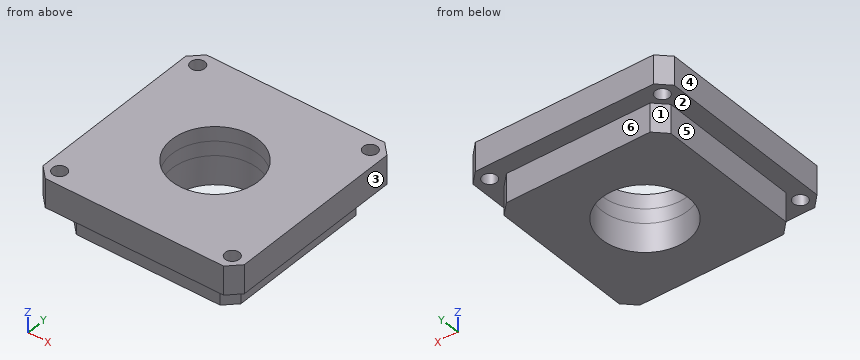
Autodesk Inventor part; units mm, degrees
ref_plane "YZ Plane" through (0, 0, 0) normal (1, 0, 0) x (0, 1, 0)
ref_plane "XZ Plane" through (0, 0, 0) normal (0, 1, 0) x (-1, 0, 0)
ref_plane "XY Plane" through (0, 0, 0) normal (0, 0, 1) x (1, 0, 0)
sketch "Sketch5" plane through (0, 0, 0) normal (0, 0, 1) x (1, 0, 0)
  circle A0 centre (15, -15) radius 1.2295
  circle A1 centre (-15, 15) radius 1.2295
  circle A2 centre (15, 15) radius 1.2295
  circle A3 centre (-15, -15) radius 1.2295
  line L0 (-15.5, -17.5) -> (-17.5, -15.5)
  line L1 (-15.5, -17.5) -> (15.5, -17.5)
  line L2 (17.5, -15.5) -> (15.5, -17.5)
  line L3 (17.5, -15.5) -> (17.5, 15.5)
  line L4 (15.5, 17.5) -> (17.5, 15.5)
  line L5 (15.5, 17.5) -> (-15.5, 17.5)
  line L6 (-17.5, 15.5) -> (-15.5, 17.5)
  line L7 (-17.5, 15.5) -> (-17.5, -15.5)
  circle A4 centre (0, 0) radius 7.5
  dimension "d59" = 15
extrude "Extrusion4" add sketch "Sketch5" against normal mid plane 5
sketch "Sketch6" plane through (0, 0, -2.5) normal (0, 0, -1) x (-1, 0, 0)
  line L0 (14.5, 12.5) -> (14.5, -12.5)
  line L1 (12.5, 14.5) -> (14.5, 12.5)
  line L2 (-12.5, 14.5) -> (12.5, 14.5)
  line L3 (-14.5, 12.5) -> (-12.5, 14.5)
  line L4 (-14.5, -12.5) -> (-14.5, 12.5)
  line L5 (-12.5, -14.5) -> (-14.5, -12.5)
  line L6 (12.5, -14.5) -> (-12.5, -14.5)
  line L7 (14.5, -12.5) -> (12.5, -14.5)
  circle A0 centre (0, 0) radius 7.5
extrude "Extrusion5" add sketch "Sketch6" along normal blind 5
properties part number "Front cover for servo motor 250 W" material "PBT Plastic"
The model under review builds one solid part; all positions refer to its coordinate system, in mm. Face numbers are marked on the shaded views. A direction names the side the tool comes from. Round coordinates to 2 decimals unless told otherwise and drop trailing zeros. Order: outer loops, then holes, each group sorted by start corner. A loop starts at its lowest first (then second) coordinate and runs counter-clockwise, first axis right, second up. Notation, with made-up numbers: (4.5, -36) -> (49.5, -36) arc R16 cw to (49.5, -27) -> close; hole circle Ø7 at (15.25, 35). An arc over 180 degrees is marked (long way). One line per item, written item: value. Start each with the question number.
Q1. Clearance check with flat-ended pins moving along their axes: pin 1 Ø2.5 at (x, z) = (4, -5.5) entering from -Y; pin 2 Ø2 at (x, y) = (-15, 15) entering from -Z; pin 3 Ø2.5 at (y, z) = (5, -4.5) entering from -X; pin 4 Ø2.5 at (x, z) = (3, -4) entering from +Y. State where each tip first meets the part, or that it passes through.
Q2. Machinability: for the marked faces 4, 5 and 6, which of the approach directions +Z, -Z, +X, -X, +Y, -Y give a long, thin tool a straight path to every point of the face, cutting with its end or side? Answer none if there is none.
Q3. Wall thickness on line 1 (Y direction, x = -15, z = 1.2); line 2 (X direction, y = 0, z = -6.4): over which ranges is each line inside the solid? List them lowest first.
Q4. Take a section at C-C (z = -5). Write out the cut boundary in (x, y).
Q5. Take a section at A-A (y = 15). Write out the cut boundary in (x, z), and give its area (3 significant figures).
Q6. Take a section at D-D (y = 0). Write out the cut boundary in (x, z), and give its area (3 significant figures).
Q7. Mouldability with a two-part tool opening along X and no side actions: class the marked faces 1, 2 and 3 as released by +X, released by -X, zero draft, split by the parting line, or undercut.
Reported:
1. pin 1: stops at y = -14.5
1. pin 2: passes through
1. pin 3: stops at x = -14.5
1. pin 4: stops at y = 14.5
2. face 4: +Z, -Z, -X, +Y, -Y
2. face 5: -Z, -X, +Y, -Y
2. face 6: -Z, +X, -X, +Y
3. line 1: y = -17.5 to -16.23, -13.77 to 13.77, 16.23 to 17.5
3. line 2: x = -14.5 to -7.5, 7.5 to 14.5
4. outline: (-14.5, -12.5) -> (-12.5, -14.5) -> (12.5, -14.5) -> (14.5, -12.5) -> (14.5, 12.5) -> (12.5, 14.5) -> (-12.5, 14.5) -> (-14.5, 12.5) -> close; hole circle Ø15 at (0, 0)
5. outline: (-17.5, -2.5) -> (-16.23, -2.5) -> (-16.23, 2.5) -> (-17.5, 2.5) -> close; (-13.77, -2.5) -> (13.77, -2.5) -> (13.77, 2.5) -> (-13.77, 2.5) -> close; (16.23, -2.5) -> (17.5, -2.5) -> (17.5, 2.5) -> (16.23, 2.5) -> close
5. area: 150 mm2
6. outline: (-17.5, -2.5) -> (-14.5, -2.5) -> (-14.5, -7.5) -> (-7.5, -7.5) -> (-7.5, 2.5) -> (-17.5, 2.5) -> close; (7.5, -7.5) -> (14.5, -7.5) -> (14.5, -2.5) -> (17.5, -2.5) -> (17.5, 2.5) -> (7.5, 2.5) -> close
6. area: 170 mm2
7. face 1: released by -X
7. face 2: zero draft
7. face 3: released by +X
